Input: part model. Units: mm. Frame: model coordinates. A direction names the side the tool comes from. Coordinates: 2 decimals unless noted, no trailing zeros. Write each loop counter-clockwise with the first axis right and the second up, starting at its lowest first coordinate (ties: lowest second). Pieces come first, ordered by that corner, then holes. Notation, with made-up numbers: (5.5, -19) -> (10.5, -19) arc R24 ccw to (10.5, 6) -> close; hole circle Ø8 at (17.5, 10.5). An arc over 180 degrees is marked (long way). Use one line per item in the form item = value. Start each with the question number.
(1) Cut plane B-B on x = 1.5. Return the cut outline in (y, z).
(2) Cut plane A-A on z = 0. Return the cut outline in (x, y), plus the area to 3 significant figures.
(3) First-contact query: pin 1 (1.5 mm diameter, centred on x = -34.5, y = 4, fed in from +Z); pin 2 (8 mm diameter, centred on x = -11, y = 9.5, fed in from -Z); pin 3 (3 mm diameter, centred on x = -29.5, y = 8.5, fed in from +Z); pin 4 (5 mm diameter, centred on x = -25, z = 13, fed in from +Y). Flat tips, straight axial feed; report the tip coordinate or a pass-through.
(4) Cut plane D-D on y = 12.75. Return the cut outline in (x, z).
(5) Cut plane C-C on z = -16. Return the cut outline in (x, y).
(6) Pull-direction query (Z, two-part tool) for faces 1 (the face through (-19, 15, 11)), 2 (the face through (3, 7, 0)), 3 (the face through (-16.3, 7.4, 27.47)); classes: released by +Z, released by -Z, zero draft, split by the parting line, or undercut.
(7) Set-up query: faces 4 (the face through (-43, 7, -48)), 5 (the face through (-27.97, 7.4, 18.51)). Return all of +Z, -Z, +X, -X, +Y, -Y with unobstructed straight access to the full face (end or side cutting, diameter ignored); none if empty.
(8) Ray query, line 1 along Z through (x, y) = (0, 10.75); line 2 along Z through (x, y) = (3.5, 13.25); line 3 along X through (y, z) = (1.5, 26). Return the intervals inside material, ascending.
Autodesk Inventor part; units mm, degrees
ref_plane "YZ Plane" through (0, 0, 0) normal (1, 0, 0) x (0, 1, 0)
ref_plane "XZ Plane" through (0, 0, 0) normal (0, 1, 0) x (-1, 0, 0)
ref_plane "XY Plane" through (0, 0, 0) normal (0, 0, 1) x (1, 0, 0)
sketch "Sketch1" plane through (0, 0, 0) normal (0, 1, 0) x (-1, 0, 0)
  circle A0 centre (0, 0) radius 3
  circle A1 centre (0, 0) radius 8.75
  line L0 (0, 0) -> (48, 0) construction
  line L1 (48, 48) -> (48, -48) construction
  line L2 (48, 48) -> (38, 48)
  line L3 (38, 48) -> (38, 28)
  line L4 (38, 28) -> (48, 28)
  line L5 (48, 28) -> (48, 48)
  line L6 (38, 48) -> (-6.0137, 6.3559)
  line L7 (38, 28) -> (17.6546, 8.75)
  line L8 (17.6546, 8.75) -> (17.6546, 0)
  line L9 (48, -48) -> (38, -48)
  line L10 (38, -48) -> (38, -28)
  line L11 (38, -28) -> (48, -28)
  line L12 (48, -28) -> (48, -48)
  line L13 (38, -48) -> (-6.0137, -6.3559)
  line L14 (38, -28) -> (17.6546, -8.75)
  line L15 (17.6546, -8.75) -> (17.6546, 0)
  line L16 (48, 28) -> (38, 28)
  line L17 (38, 28) -> (38, -28)
  line L18 (38, -28) -> (48, -28)
  line L19 (48, -28) -> (48, 28)
  dimension "d1" = 17.5
  dimension "d0" = 6
  dimension "d2" = 48
  dimension "d3" = 96
  dimension "d4" = 10
  dimension "d5" = 20
  dimension "d6" = 17.5
extrude "Extrusion1" add sketch "Sketch1" along normal blind 15 contours A1 | A1 L6 L3 L7 L8 L15 L14 L10 L13 | L2 L5 L4 L3 | L10 L11 L12 L9 | L4 L19 L11 L17
ref_plane "Work Plane1" through (0.0004, 0, -8.75) normal (-1, 0, 0) x (0, 0, 1)
properties part number "Custom Wheel Mount"
Values:
q1.outline = (0, -10.63) -> (15, -10.63) -> (15, -2.6) -> (0, -2.6) -> close; (0, 2.6) -> (15, 2.6) -> (15, 10.63) -> (0, 10.63) -> close
q2.outline = (-48, 0) -> (-38, 0) -> (-38, 15) -> (-48, 15) -> close; (-17.65, 0) -> (-3, 0) -> (-3, 15) -> (-17.65, 15) -> close; (3, 0) -> (8.75, 0) -> (8.75, 15) -> (3, 15) -> close
q2.area = 456 mm2
q3.pin_1 = 45.4
q3.pin_2 = -26.24
q3.pin_3 = 41.38
q3.pin_4 = 15
q4.outline = (-48, -48) -> (-38, -48) -> (6.01, -6.36) arc R8.75 ccw to (6.01, 6.36) -> (-38, 48) -> (-48, 48) -> close; hole (-38, -28) -> (-17.65, -8.75) -> (-17.65, 8.75) -> (-38, 28) -> close; hole circle Ø6 at (0, 0)
q5.outline = (-48, 0) -> (-38, 0) -> (-38, 15) -> (-48, 15) -> close; (-25.32, 0) -> (-4.18, 0) -> (-4.18, 15) -> (-25.32, 15) -> close
q6.face_1 = zero draft
q6.face_2 = undercut
q6.face_3 = released by +Z
q7.face_4 = -Z, +X, -X, +Y, -Y
q7.face_5 = +Y, -Y
q8.line_1 = -12.05 to -3, 3 to 12.05
q8.line_2 = -8.73 to 8.73
q8.line_3 = -48 to -38, -35.89 to -14.75
